from build123d import *

# Parameters (mm, degrees)
F1_W      = 41.5
F1_H      = 42.2
F2_DEPTH  = 10
F0_W      = 31.5
F0_H      = 32.2
F3_DEPTH  = 25
F4_W      = 5
F4_H      = 10
F5_DEPTH  = 10
F6_W      = 71
F6_H      = 10
F7_DEPTH  = 5
F8_W      = 5
F8_H      = 10
F9_DEPTH  = 25
F11_R     = 3.75
F12_DEPTH = 3
F13_W     = 31.5
F13_H     = 10
F14_DEPTH = 10
F10_R     = 3.75
F15_DEPTH = 3


with BuildPart() as f2:
    # F1 (on Front) → F2 (new body)
    with BuildSketch(Plane.XZ):
        with Locations((-15.75, 16.1)):
            Rectangle(F1_W, F1_H)
    extrude(amount=F2_DEPTH)

    # F0 (on Front) → F3 (cut)
    with BuildSketch(Plane.XZ):
        with Locations((-15.75, 16.1)):
            Rectangle(F0_W, F0_H)
    extrude(amount=F3_DEPTH, mode=Mode.SUBTRACT)

    # F4 (on face) → F5 (join)
    with BuildSketch(Plane(origin=(0, 0, -5), x_dir=(1, 0, 0), z_dir=(0, 0, -1))):
        with Locations((2.5, 5)):
            Rectangle(F4_W, F4_H)
        with Locations((-34, 5)):
            Rectangle(F4_W, F4_H)
    extrude(amount=F5_DEPTH)

    # F6 (on face) → F7 (join)
    with BuildSketch(Plane(origin=(0, 0, -15), x_dir=(1, 0, 0), z_dir=(0, 0, -1))):
        with Locations((-15.75, 5)):
            Rectangle(F6_W, F6_H)
    extrude(amount=F7_DEPTH)

    # F8 (on face) → F9 (join)
    with BuildSketch(Plane(origin=(0, 0, -20), x_dir=(1, 0, 0), z_dir=(0, 0, -1))):
        with Locations((17.25, 5)):
            Rectangle(F8_W, F8_H)
        with Locations((-48.75, 5)):
            Rectangle(F8_W, F8_H)
    extrude(amount=F9_DEPTH)

    # F11 (on face) → F12 (join)
    with BuildSketch(Plane.YZ.offset(-46.25)):
        with Locations((-5, -40)):
            Circle(F11_R)
    extrude(amount=F12_DEPTH)

    # F13 (on face) → F14 (join)
    with BuildSketch(Plane(origin=(0, 0, 0), x_dir=(-1, 0, 0), z_dir=(0, 1, 0))):
        with Locations((15.75, -10)):
            Rectangle(F13_W, F13_H)
    extrude(amount=-F14_DEPTH)

    # F10 (on face) → F15 (join)
    with BuildSketch(Plane(origin=(14.75, 0, 0), x_dir=(0, -1, 0), z_dir=(-1, 0, 0))):
        with Locations((5, -40)):
            Circle(F10_R)
    extrude(amount=F15_DEPTH)


solid = f2.part
Model file for the job. Use its own axes, mm. A direction names the side the tool comes from. Coordinates: 2 decimals unless noted, no trailing zeros. Order: outer loops, then holes, each group sorted by start corner. A loop starts at its lowest first (then second) coordinate and runs counter-clockwise, first axis right, second up. Notation, with made-up numbers: M 81.5,73 L 103.5,73 A8 cw 103.5,80 Z; hole C 27,43.5 d6. An arc over 180 degrees is marked long. Return JSON: item names as keys, results as strings.
1. Saw through at A-A (x = -7.5). Give the cut face in (y, z).
Ans:
{"outline": "M -10,-20 L 0,-20 L 0,0 L -10,0 Z; M -10,32.2 L 0,32.2 L 0,37.2 L -10,37.2 Z"}
2. Tool access for faces 1 (the face through (-43.25, -5, -40)), 2 (the face through (-16, -5, 0)), 3 (the face through (-36.5, -5, 11)): list every direction of +Z, -Z, +X, -X, +Y, -Y with a clear straight run to the whole face (end or side of a thin tool).
Ans:
{"face 1": "-Z, +Y, -Y", "face 2": "+Y, -Y", "face 3": "+Z, -X, +Y, -Y"}
3. Flat gauge pins, fed straight in: pin 1 (2 mm diameter, centred on x = -39, y = -2.5, fed in from -Z); pin 2 (5 mm diameter, centred on y = -2.5, z = 6, fed in from +X); pin 3 (1 mm diameter, centred on x = -43, y = -9, fed in from +Z); pin 4 (3 mm diameter, centred on x = 4.5, z = -22.5, fed in from +Y). Where does each tip first touch, or does it go through?
Ans:
{"pin 1": "z = -20", "pin 2": "x = 5", "pin 3": "z = -15", "pin 4": "through"}
4. Drill centre lines: probe 1 along Z at (x, y) = (-5, -4.75); probe 2 along X at (y, z) = (-6.5, -31.5); probe 3 along X at (y, z) = (-4.5, 22). Where is each one in solid material? Low to high.
Ans:
{"probe 1": "-20 to 0, 32.2 to 37.2", "probe 2": "-51.25 to -46.25, 14.75 to 19.75", "probe 3": "-36.5 to -31.5, 0 to 5"}
5. Saw through at D-D (z = -4). Give the cut face in (x, y), and give its area (3 significant figures).
Ans:
{"outline": "M -36.5,-10 L 5,-10 L 5,0 L -36.5,0 Z", "area": "415 mm^2"}
6. Saw through at C-C (y = -5). Give the cut face in (x, z).
Ans:
{"outline": "M -51.25,-45 L -46.25,-45 L -46.25,-43.75 L -43.25,-43.75 L -43.25,-36.25 L -46.25,-36.25 L -46.25,-20 L 14.75,-20 L 14.75,-36.25 L 11.75,-36.25 L 11.75,-43.75 L 14.75,-43.75 L 14.75,-45 L 19.75,-45 L 19.75,-15 L 5,-15 L 5,37.2 L -36.5,37.2 L -36.5,-15 L -51.25,-15 Z; hole M -31.5,0 L 0,0 L 0,32.2 L -31.5,32.2 Z"}
7. Pull direction Z, two halves, no side cores. Call faces 4 (the face through (12, -5, -15)), 5 (the face through (19.75, -5, -30)), 6 (the face through (14.75, -5, -30)): +Z half, -Z half, draft (parallel to the pull), parting line (faces both ways), or undercut.
Ans:
{"face 4": "+Z half", "face 5": "draft", "face 6": "undercut"}
8. Saw through at B-B (z = -40). Give the cut face in (x, y).
Ans:
{"outline": "M -51.25,-10 L -46.25,-10 L -46.25,-8.75 L -43.25,-8.75 L -43.25,-1.25 L -46.25,-1.25 L -46.25,0 L -51.25,0 Z; M 11.75,-8.75 L 14.75,-8.75 L 14.75,-10 L 19.75,-10 L 19.75,0 L 14.75,0 L 14.75,-1.25 L 11.75,-1.25 Z"}
